The listing builds one solid part. Answer for the finished solid, in the listing's coordinates (mm). Coordinates: 2 decimals unless noted, no trailing zeros. Order: outer loops, then holes, each group sorted by start corner. A loop starts at its lowest first (then second) coordinate and runs counter-clockwise, first axis right, second up. Notation, with made-up numbers: M 51.5,69.5 L 102.5,69.5 A18 cw 102.5,92.5 Z; hole C -38.5,33.5 d4. An arc over 180 degrees is marked long. One line per item, written item: value. Start each with the question number.
Q1. The part is cut by section A-A on x = -8. Give the vertices of the cut face in (y, z).
Q2. Straight lines are drawn through the part: line 1 along Z through (x, y) = (-33, 1.8) (3 decimals); line 2 along X through (y, z) = (3, -10); line 3 along Z through (x, y) = (-140, 3.65). For each, find the intervals that lie inside material, in ascending order. Write a range as [from, to].
Q3. The part is cut by section D-D on x = -138.5. Give the vertices of the cut face in (y, z).
Q4. The part is cut by section B-B on y = 3.2. Give the vertices of the cut face in (x, z) (3 decimals).
Q5. The part is cut by section C-C on z = -24. Give the vertices of the cut face in (x, y).
Q6. Each of these flat-tipped pins is pushed along its axis until it touches: pin 1 Ø1.7 at (y, z) = (2.5, -0.5) entering from +X; pin 2 Ø0.5 at (y, z) = (3.5, -1) entering from -X; pin 3 Ø2.5 at (x, y) = (-95.5, 3.5) entering from -Z. Where does it stop, or does it pass through?
Autodesk Inventor part; units mm, degrees
ref_plane "YZ Plane" through (0, 0, 0) normal (1, 0, 0) x (0, 1, 0)
ref_plane "XZ Plane" through (0, 0, 0) normal (0, 1, 0) x (-1, 0, 0)
ref_plane "XY Plane" through (0, 0, 0) normal (0, 0, 1) x (1, 0, 0)
sketch "草图1" plane through (0, 0, 0) normal (0, 1, 0) x (-1, 0, 0)
  line L0 (0, 0) -> (140, 0)
  line L1 (140, 0) -> (140, -22)
  line L2 (140, -22) -> (0, -22)
  line L3 (0, -22) -> (0, 0)
  circle A0 centre (100, -11) radius 11
  circle A1 centre (100, -11) radius 4.15
  circle A2 centre (140, -11) radius 11
  circle A3 centre (140, -11) radius 4.15
  line L4 (25, -8) -> (0, -8)
  line L5 (0, -8) -> (0, -21)
  line L6 (0, -21) -> (25, -21)
  line L7 (25, -21) -> (25, -8)
  line L8 (32, -22) -> (0, -22)
  line L9 (0, -22) -> (0, -29)
  line L10 (0, -29) -> (32, -29)
  line L11 (32, -29) -> (32, -22)
  line L12 (32, -22) -> (25, -29)
  circle A4 centre (8, -1.55) radius 1.55
  line L13 (9.55, 0) -> (6.45, 0)
  line L14 (6.45, 0) -> (6.45, -1.55)
  line L15 (6.45, -1.55) -> (9.55, -1.55)
  line L16 (9.55, -1.55) -> (9.55, 0)
  circle A5 centre (33, -14.5) radius 1.525
  line L17 (25, -14.5) -> (20.7418, -14.5)
  circle A6 centre (41, -14.5) radius 1.525
  circle A7 centre (8, -27.45) radius 1.55
  line L18 (6.45, -27.45) -> (9.55, -27.45)
  line L19 (9.55, -27.45) -> (9.55, -29)
  line L20 (9.55, -29) -> (6.45, -29)
  line L21 (6.45, -29) -> (6.45, -27.45)
  point P0 (9.55, -1.55)
  point P1 (6.45, 0)
  point P2 (0, -8)
  point P3 (6.45, -29)
  dimension "d11" = 3.1
  dimension "d17" = 3.1
  dimension "d0" = 22
  dimension "d1" = 140
  dimension "d2" = 100
  dimension "d3" = 8.3
  dimension "d4" = 8.3
  dimension "d5" = 13
  dimension "d6" = 8
  dimension "d7" = 8
  dimension "d8" = 45
  dimension "d9" = 25
  dimension "d10" = 32
  dimension "d12" = 3.05
  dimension "d13" = 8
  dimension "d14" = 3.05
  dimension "d15" = 8
  dimension "d16" = 8
extrude "拉伸1" add sketch "草图1" along normal blind 5 contours L0 L14 A4 L16 A0 L2 L3 L6 L7 L4 | L2 L12 L10 L19 A7 L21 L9 | L0 A2 L2 A0 | A0 | A2 L1 A3 | L1 A3 A2
chamfer "倒角1" distance 2 angle 45 4 edges at (0, 2.5, 0) (-25, 2.5, -21) (0, 2.5, -29) (-25, 2.5, -8)
chamfer "倒角2" distance 0.5 angle 45 2 edges at (0, 2.5, -8) (0, 2.5, -21)
properties part number "leg2"
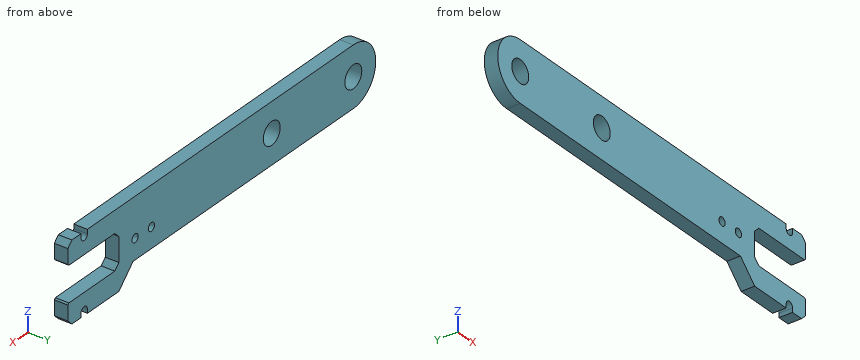
Output:
1. outline: M 0,-25.9 L 5,-25.9 L 5,-21 L 0,-21 Z; M 0,-8 L 5,-8 L 5,-3.1 L 0,-3.1 Z
2. line 1: z = [-22, -16.025], [-12.975, 0]
2. line 2: x = [-150.95, -144.03], [-135.97, -104.03], [-95.97, -25]
2. line 3: z = [-22, -15.15], [-6.85, 0]
3. outline: M 0,-22 L 5,-22 L 5,-14.87 L 0,-14.87 Z; M 0,-7.13 L 5,-7.13 L 5,0 L 0,0 Z
4. outline: M -140,-22 L -32,-22 L -25,-29 L -9.55,-29 L -9.55,-27.45 A1.55 cw -6.45,-27.45 L -6.45,-29 L -2,-29 L 0,-27 L 0,-21.5 L -0.5,-21 L -23,-21 L -25,-19 L -25,-10 L -23,-8 L -0.5,-8 L 0,-7.5 L 0,-2 L -2,0 L -6.45,0 L -6.45,-1.55 A1.55 cw -9.55,-1.55 L -9.55,0 L -140,0 A11 ccw Z; hole C -140,-11 d8.3; hole C -100,-11 d8.3; hole C -41,-14.5 d3.05; hole C -33,-14.5 d3.05
5. outline: M -30,0 L 0,0 L 0,5 L -30,5 Z
6. pin 1: stops at x = -0.65
6. pin 2: stops at x = -145.09
6. pin 3: stops at z = -22
